```python
from build123d import *

# Parameters (mm, degrees)
F1_DEPTH = 25.4
F2_DEPTH = 25.4
F3_DEPTH = 25.4


with BuildPart() as f1:
    # F0 (on Front) → F1 (new body)
    with BuildSketch(Plane.XZ):
        with BuildLine():
            ThreePointArc((-32.6936654747, 64.7734031081), (-48.13655305, 49.9296563149), (-68.8628588319, 44.5222683907))
            Line((-68.8628588319, 44.5222683907), (58.1371411681, 44.5222683907))
            Line((58.1371411681, 44.5222683907), (22.5408878177, 64.7734031081))
            Line((22.5408878177, 64.7734031081), (-32.6936654747, 64.7734031081))
        make_face()
        with BuildLine():
            Line((58.1371411681, 44.5222683907), (-68.8628588319, 44.5222683907))
            Line((-68.8628588319, 44.5222683907), (-68.8628588319, 19.1222683907))
            Line((-68.8628588319, 19.1222683907), (-56.3345537444, 19.1222683907))
            ThreePointArc((-56.3345537444, 19.1222683907), (-48.1413485784, 36.0579067807), (-33.43944267, 24.3191495538))
            ThreePointArc((-33.43944267, 24.3191495538), (-33.7380519171, 21.6546101194), (-34.6190645437, 19.1222683907))
            Line((-34.6190645437, 19.1222683907), (55.7402772585, 19.1222683907))
            ThreePointArc((55.7402772585, 19.1222683907), (54.7678046883, 26.416830746), (58.1371411681, 32.9593008102))
            Line((58.1371411681, 32.9593008102), (58.1371411681, 44.5222683907))
        make_face()
    extrude(amount=F1_DEPTH)

    # F0 (on Front) → F2 (join)
    with BuildSketch(Plane.XZ):
        with BuildLine():
            ThreePointArc((-32.6936654747, 64.7734031081), (-48.13655305, 49.9296563149), (-68.8628588319, 44.5222683907))
            Line((-68.8628588319, 44.5222683907), (58.1371411681, 44.5222683907))
            Line((58.1371411681, 44.5222683907), (22.5408878177, 64.7734031081))
            Line((22.5408878177, 64.7734031081), (-32.6936654747, 64.7734031081))
        make_face()
        with BuildLine():
            Line((58.1371411681, 44.5222683907), (-68.8628588319, 44.5222683907))
            Line((-68.8628588319, 44.5222683907), (-68.8628588319, 19.1222683907))
            Line((-68.8628588319, 19.1222683907), (-56.3345537444, 19.1222683907))
            ThreePointArc((-56.3345537444, 19.1222683907), (-48.1413485784, 36.0579067807), (-33.43944267, 24.3191495538))
            ThreePointArc((-33.43944267, 24.3191495538), (-33.7380519171, 21.6546101194), (-34.6190645437, 19.1222683907))
            Line((-34.6190645437, 19.1222683907), (55.7402772585, 19.1222683907))
            ThreePointArc((55.7402772585, 19.1222683907), (54.7678046883, 26.416830746), (58.1371411681, 32.9593008102))
            Line((58.1371411681, 32.9593008102), (58.1371411681, 44.5222683907))
        make_face()
        with BuildLine():
            Line((97.3853468895, 40.5878610909), (58.1371411681, 44.5222683907))
            Line((58.1371411681, 44.5222683907), (58.1371411681, 32.9593008102))
            ThreePointArc((58.1371411681, 32.9593008102), (71.5481129353, 35.6873436348), (79.1678599605, 24.3191495538))
            ThreePointArc((79.1678599605, 24.3191495538), (78.8761964322, 21.6575453897), (78.0150490125, 19.1222683907))
            Line((78.0150490125, 19.1222683907), (97.3853468895, 19.1222683907))
            Line((97.3853468895, 19.1222683907), (97.3853468895, 23.5926117748))
            Line((97.3853468895, 23.5926117748), (97.3853468895, 40.5878610909))
        make_face()
        with BuildLine():
            ThreePointArc((79.1678599605, 24.3191495538), (71.5481129353, 35.6873436348), (58.1371411681, 32.9593008102))
            Line((58.1371411681, 32.9593008102), (58.1371411681, 19.1222683907))
            Line((58.1371411681, 19.1222683907), (78.0150490125, 19.1222683907))
            ThreePointArc((78.0150490125, 19.1222683907), (78.8761964322, 21.6575453897), (79.1678599605, 24.3191495538))
        make_face()
        with BuildLine():
            Line((58.1371411681, 19.1222683907), (58.1371411681, 32.9593008102))
            ThreePointArc((58.1371411681, 32.9593008102), (54.7678046883, 26.416830746), (55.7402772585, 19.1222683907))
            Line((55.7402772585, 19.1222683907), (58.1371411681, 19.1222683907))
        make_face()
        with BuildLine():
            ThreePointArc((-33.43944267, 24.3191495538), (-48.1413485784, 36.0579067807), (-56.3345537444, 19.1222683907))
            Line((-56.3345537444, 19.1222683907), (-34.6190645437, 19.1222683907))
            ThreePointArc((-34.6190645437, 19.1222683907), (-33.7380519171, 21.6546101194), (-33.43944267, 24.3191495538))
        make_face()
        with BuildLine():
            Line((-34.6190645437, 19.1222683907), (-56.3345537444, 19.1222683907))
            ThreePointArc((-56.3345537444, 19.1222683907), (-45.476809144, 12.2817830798), (-34.6190645437, 19.1222683907))
        make_face()
        with BuildLine():
            Line((78.0150490125, 19.1222683907), (58.1371411681, 19.1222683907))
            Line((58.1371411681, 19.1222683907), (55.7402772585, 19.1222683907))
            ThreePointArc((55.7402772585, 19.1222683907), (66.8776631355, 12.0289527288), (78.0150490125, 19.1222683907))
        make_face()
    extrude(amount=F2_DEPTH)

    # F0 (on Front) → F3 (join)
    with BuildSketch(Plane.XZ):
        with BuildLine():
            Line((97.3853468895, 40.5878610909), (58.1371411681, 44.5222683907))
            Line((58.1371411681, 44.5222683907), (58.1371411681, 32.9593008102))
            ThreePointArc((58.1371411681, 32.9593008102), (71.5481129353, 35.6873436348), (79.1678599605, 24.3191495538))
            ThreePointArc((79.1678599605, 24.3191495538), (78.8761964322, 21.6575453897), (78.0150490125, 19.1222683907))
            Line((78.0150490125, 19.1222683907), (97.3853468895, 19.1222683907))
            Line((97.3853468895, 19.1222683907), (97.3853468895, 23.5926117748))
            Line((97.3853468895, 23.5926117748), (97.3853468895, 40.5878610909))
        make_face()
        with BuildLine():
            ThreePointArc((79.1678599605, 24.3191495538), (71.5481129353, 35.6873436348), (58.1371411681, 32.9593008102))
            Line((58.1371411681, 32.9593008102), (58.1371411681, 19.1222683907))
            Line((58.1371411681, 19.1222683907), (78.0150490125, 19.1222683907))
            ThreePointArc((78.0150490125, 19.1222683907), (78.8761964322, 21.6575453897), (79.1678599605, 24.3191495538))
        make_face()
    extrude(amount=F3_DEPTH)


solid = f1.part
```
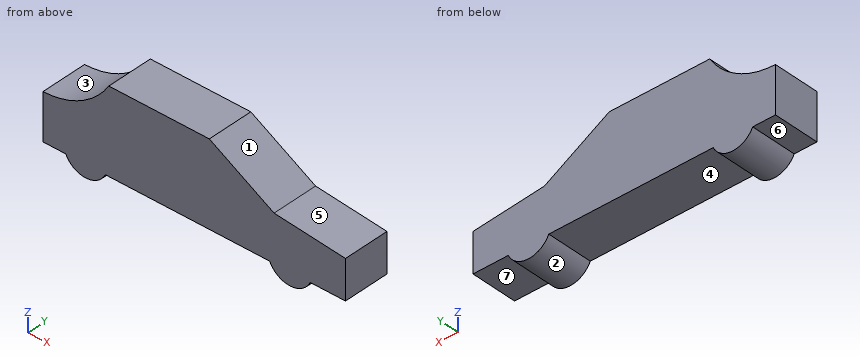
Verification items for the finished model (mm, model axes). Face numbers are marked on the shaded views. A direction names the side the tool comes from. Round coordinates to 2 decimals unless told otherwise and drop trailing zeros. Write each loop counter-clockwise with the first axis right and the second up, starting at its lowest first coordinate (ties: lowest second). Pieces come first, ordered by that corner, then holes.
1. Draft check along X on the marked faces 1, 2, 3 and 4. Enter one of: +X half, -X half, draft (parallel to the pull), parting line (faces both ways), or undercut.
2. Scan lines: L1, parallel to Z at x = 1, y = -19; L2, parallel to Z at x = 59, y = -20.5; L3, parallel to X at y = -20, z = 59. Record each from-to range of solid material in increasing order.
3. Access from +Z, -Z, +X, -X, +Y, -Y to the whole of each face (thin tool, end or side, straight path). Record for the marked faces 5, 6 and 7.
4. Section check A-A on y = -15. Enter the section's corners in (x, z).
5. Section check C-C on z = 58. Enter the section's corners in (x, y), plus the area to 3 significant figures.
6. Section check B-B on x = 84. Enter the section's corners in (y, z).
7. Gauge pin test, flat ends, axial feed: P1, Ø3, axis at y = -3, z = 17.5, coming from the -X side; P2, Ø6, axis at x = 84, y = -18, coming from the -Z side. Record the tip position at first contact, or that the pin passes through.
Answer:
1. face 1: +X half
1. face 2: undercut
1. face 3: -X half
1. face 4: undercut
2. L1: z = 19.12 to 64.77
2. L2: z = 14.89 to 44.44
2. L3: x = -36.94 to 32.69
3. face 5: +Z, +X, +Y, -Y
3. face 6: -Z, -X, +Y, -Y
3. face 7: -Z, +X, +Y, -Y
4. outline: (-68.86, 19.12) - (-56.33, 19.12) arc R12.04 ccw to (-34.62, 19.12) - (55.74, 19.12) arc R12.29 ccw to (78.02, 19.12) - (97.39, 19.12) - (97.39, 40.59) - (58.14, 44.52) - (22.54, 64.77) - (-32.69, 64.77) arc R42.43 cw to (-68.86, 44.52) - close
5. outline: (-37.85, -25.4) - (34.45, -25.4) - (34.45, 0) - (-37.85, 0) - close
5. area: 1,840 mm2
6. outline: (-25.4, 19.12) - (0, 19.12) - (0, 41.93) - (-25.4, 41.93) - close
7. P1: stops at x = -56.28
7. P2: stops at z = 19.12
